```python
from build123d import *

# Parameters (mm, degrees)
SKETCH_1_W          = 10
SKETCH_1_H          = 10
SKETCH_1_W_2        = 8
SKETCH_1_H_2        = 8
EXTRUDE_1_DEPTH     = 50
CUT_EXTRUDE_1_REACH = 53.962
SKETCH_2_R          = 2.1


with BuildPart() as part:
    # ｽｹｯﾁ1 → 押し出し-薄板1 (new body)
    with BuildSketch(Plane.XY):
        with Locations((5, 5)):
            Rectangle(SKETCH_1_W, SKETCH_1_H)
        with Locations((5, 5)):
            Rectangle(SKETCH_1_W_2, SKETCH_1_H_2, mode=Mode.SUBTRACT)
    extrude(amount=EXTRUDE_1_DEPTH)

    # ｶｯﾄ - 押し出し1: up to this face of the body (flat: up to its plane)
    cut_extrude_1_end = Plane(part.part.faces().sort_by_distance((0, 5, 25))[0])
    # ｽｹｯﾁ2 → ｶｯﾄ - 押し出し1 (cut, up to the picked face)
    with BuildSketch(Plane(origin=(10, 0, 0), x_dir=(0, 0, -1), z_dir=(1, 0, 0)), mode=Mode.PRIVATE) as cut_extrude_1_sk1:
        with Locations((-5, 5)):
            Circle(SKETCH_2_R)
    cut_extrude_1_tool1 = split(extrude(cut_extrude_1_sk1.sketch, amount=-CUT_EXTRUDE_1_REACH, mode=Mode.PRIVATE), bisect_by=cut_extrude_1_end, keep=Keep.BOTH, mode=Mode.PRIVATE)
    # ｽｹｯﾁ2 → ｶｯﾄ - 押し出し1 (cut, up to the picked face)
    with BuildSketch(Plane(origin=(10, 0, 0), x_dir=(0, 0, -1), z_dir=(1, 0, 0)), mode=Mode.PRIVATE) as cut_extrude_1_sk2:
        with Locations((-15, 5)):
            Circle(SKETCH_2_R)
    cut_extrude_1_tool2 = split(extrude(cut_extrude_1_sk2.sketch, amount=-CUT_EXTRUDE_1_REACH, mode=Mode.PRIVATE), bisect_by=cut_extrude_1_end, keep=Keep.BOTH, mode=Mode.PRIVATE)
    # ｽｹｯﾁ2 → ｶｯﾄ - 押し出し1 (cut, up to the picked face)
    with BuildSketch(Plane(origin=(10, 0, 0), x_dir=(0, 0, -1), z_dir=(1, 0, 0)), mode=Mode.PRIVATE) as cut_extrude_1_sk3:
        with Locations((-45, 5)):
            Circle(SKETCH_2_R)
    cut_extrude_1_tool3 = split(extrude(cut_extrude_1_sk3.sketch, amount=-CUT_EXTRUDE_1_REACH, mode=Mode.PRIVATE), bisect_by=cut_extrude_1_end, keep=Keep.BOTH, mode=Mode.PRIVATE)
    add(cut_extrude_1_tool1.solids().sort_by(Axis((10, 5, 5), (-1, 0, 0)))[0], mode=Mode.SUBTRACT)
    add(cut_extrude_1_tool2.solids().sort_by(Axis((10, 5, 15), (-1, 0, 0)))[0], mode=Mode.SUBTRACT)
    add(cut_extrude_1_tool3.solids().sort_by(Axis((10, 5, 45), (-1, 0, 0)))[0], mode=Mode.SUBTRACT)


solid = part.part
```
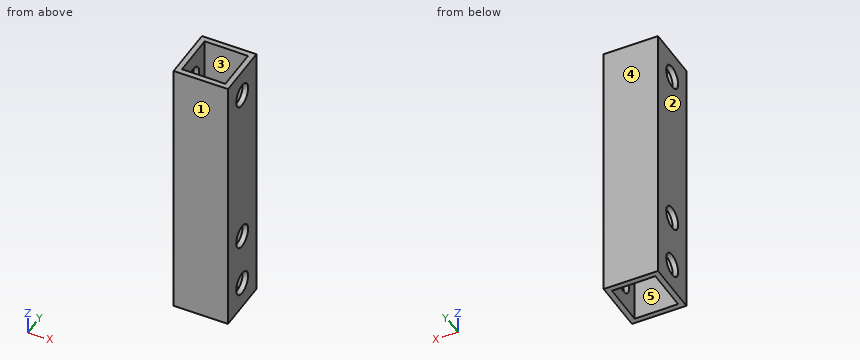
The model under review builds one solid part; all positions refer to its coordinate system, in mm. Face numbers are marked on the shaded views. A direction names the side the tool comes from. Give positions to 0.01 mm unless a question says otherwise; leave off trailing zeros. Order: outer loops, then holes, each group sorted by start corner. A loop starts at its lowest first (then second) coordinate and runs counter-clockwise, first axis right, second up. Notation, with made-up numbers: (73.25, 76.5) - (84.25, 76.5) arc R9 ccw to (84.25, 92.5) - close; hole circle Ø3 at (7.5, 81). An arc over 180 degrees is marked (long way). Use CSV: the item, a comma, the result in double quotes. Start each with the question number.
Q1. The part is to be moulded in two halves that separate along X. For the marked faces 1, 2 and 3, say which applies: +X half, -X half, draft (parallel to the pull), parting line (faces both ways), or undercut.
Q2. To check wall thickness, follow line 1 along Y through (x, z) = (0.45, 45); line 2 along Y through (x, z) = (1.75, 17.5). State the ranges of each line that lie inside material, in increasing order. Write a range as [from, to].
Q3. Clearance check with a flat-ended pin moving along its axis: pin 1 Ø3.5 at (y, z) = (5, 15) entering from -X. State where the tip first meets the part, or that it passes through.
Q4. Tool access review of the marked faces 4 and 5: name each direction out of +Z, -Z, +X, -X, +Y, -Y from which nothing blocks a thin tool from reaching the whole face with its end or side.
Q5. We need section D-D, the plane z = 37. Write out the cut boundary in (x, y).
Q6. We need section C-C, the plane z = 45. Write out the cut boundary in (x, y), and give its area (3 significant figures).
Q7. We need section A-A, the plane x = 7.5. Write out the cut boundary in (y, z), and give its area (3 significant figures).
Outcome:
1,face 1,"draft"
1,face 2,"-X half"
1,face 3,"undercut"
2,line 1,"y = [0, 2.9], [7.1, 10]"
2,line 2,"y = [0, 1], [9, 10]"
3,pin 1,"passes through"
4,face 4,"+Z, -Z, +X, -X, +Y"
4,face 5,"+Z, -Z"
5,outline,"(0, 0) - (10, 0) - (10, 10) - (0, 10) - close; hole (1, 1) - (9, 1) - (9, 9) - (1, 9) - close"
6,outline,"(0, 0) - (10, 0) - (10, 2.9) - (9, 2.9) - (9, 1) - (1, 1) - (1, 2.9) - (0, 2.9) - close; (0, 7.1) - (1, 7.1) - (1, 9) - (9, 9) - (9, 7.1) - (10, 7.1) - (10, 10) - (0, 10) - close"
6,area,"27.6 mm^2"
7,outline,"(0, 0) - (1, 0) - (1, 50) - (0, 50) - close; (9, 0) - (10, 0) - (10, 50) - (9, 50) - close"
7,area,"100 mm^2"
